```python
from build123d import *

# Parameters (mm, degrees)
SKETCH_1_R          = 14.75
EXTRUDE_1_DEPTH     = 4.2
SKETCH_2_R          = 10
EXTRUDE_2_DEPTH     = 10
SKETCH_3_R          = 7
CUT_EXTRUDE_1_DEPTH = 15.2
CHAMFER_1_SIZE      = 1


with BuildPart() as part:
    # 草图1 → 凸台-拉伸1 (new body)
    with BuildSketch(Plane.XY):
        Circle(SKETCH_1_R)
    extrude(amount=EXTRUDE_1_DEPTH)

    # 草图2 → 凸台-拉伸2 (add)
    with BuildSketch(Plane.XY.offset(4.2)):
        Circle(SKETCH_2_R)
    extrude(amount=EXTRUDE_2_DEPTH)

    # 草图3 → 切除-拉伸1 (cut, through all)
    with BuildSketch(Plane.XY.offset(14.2)):
        Circle(SKETCH_3_R)
    extrude(amount=-CUT_EXTRUDE_1_DEPTH, mode=Mode.SUBTRACT)

    # 倒角1
    chamfer_1_edges = [part.edges().sort_by_distance(p)[0] for p in [
        (-14.75, 0, 4.2),
        (-10, 0, 14.2),
    ]]
    chamfer(chamfer_1_edges, length=CHAMFER_1_SIZE)


solid = part.part
```
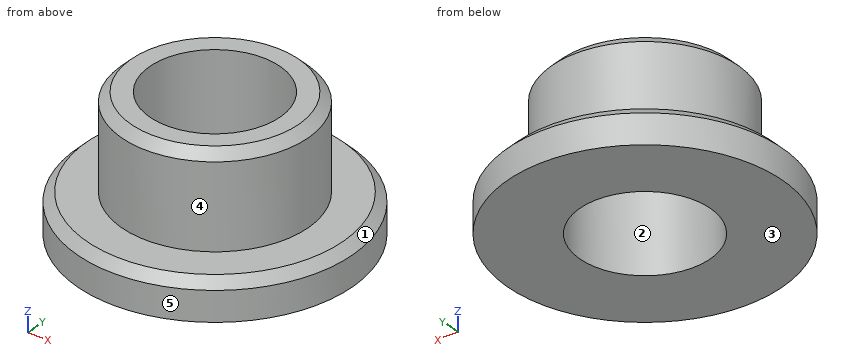
Design review of the part built by this model. Coordinates are the model's own, in mm. Face numbers are marked on the shaded views. A direction names the side the tool comes from. Coordinates: 2 decimals unless noted, no trailing zeros. Loops run counter-clockwise (first coordinate to the right, second up) from the corner with the lowest first, then second, coordinate; pieces in that order, holes last.
Q1. The part is to be moulded in two halves that separate along Y. For the marked faces 1, 2 and 3, say which applies: +Y half, -Y half, draft (parallel to the pull), parting line (faces both ways), or undercut.
Reported:
face 1: parting line
face 2: undercut
face 3: draft
Q2. We need section C-C on z = 5.75. State the section outline as (x, y) points, and give its area (3 significant figures).
Reported:
outline: circle Ø20 at (0, 0); hole circle Ø14 at (0, 0)
area: 160 mm2
Q3. For pin 1 (8 mm diameter, centred on y = -11.5, z = 6, fed in from +X); pin 2 (6 mm diameter, centred on y = -4.5, z = 10.5, fed in from -X); pin 3 (3 mm diameter, centred on y = 9.5, z = 10.5, fed in from +X), all flat-tipped, find the tip position at first contact; note any pin that passes through.
Reported:
pin 1: stops at x = 11.95
pin 2: stops at x = -9.89
pin 3: stops at x = 6
Q4. To check wall thickness, follow line 1 (Y direction, x = 0, z = 11); line 2 (Y direction, x = -4.5, z = 6.25); line 3 (X direction, y = -1, z = 10.5). State the ranges of each line that lie inside material, in increasing order.
Reported:
line 1: y = -10 to -7, 7 to 10
line 2: y = -8.93 to -5.36, 5.36 to 8.93
line 3: x = -9.95 to -6.93, 6.93 to 9.95
Q5. We need section A-A on x = 0. State the section outline as (y, z) points.
Reported:
outline: (-14.75, 0) - (-7, 0) - (-7, 14.2) - (-9, 14.2) - (-10, 13.2) - (-10, 4.2) - (-13.75, 4.2) - (-14.75, 3.2) - close; (7, 0) - (14.75, 0) - (14.75, 3.2) - (13.75, 4.2) - (10, 4.2) - (10, 13.2) - (9, 14.2) - (7, 14.2) - close
Q6. Tool access review of the marked faces 4 and 5: name each direction out of +Z, -Z, +X, -X, +Y, -Y from which nothing blocks a thin tool from reaching the whole face with its end or side.
Reported:
face 4: +Z
face 5: +Z, -Z
